The listing builds one solid part. Answer for the finished solid, in the listing's coordinates (mm). A direction names the side the tool comes from. Coordinates: 2 decimals unless noted, no trailing zeros. Order: outer loops, then holes, each group sorted by start corner. A loop starts at its lowest first (then second) coordinate and runs counter-clockwise, first axis right, second up. Notation, with made-up numbers: (52.25, 6.5) -> (70.25, 6.5) arc R21 cw to (70.25, 36.5) -> close; hole circle Ø5 at (-13.5, 32.25). An arc over 180 degrees is marked (long way). Return JSON: item names as keys, results as strings.
```python
from build123d import *
from build123d.topology import SkipClean

# Parameters (mm, degrees)
SALIENTE_EXTRUIR1_DEPTH = 2
SALIENTE_EXTRUIR2_DEPTH = 6.5
SALIENTE_EXTRUIR4_DEPTH = 2.4
SALIENTE_EXTRUIR5_START = 2.4
SALIENTE_EXTRUIR5_DEPTH = 0.9
REDONDEO1_R             = 3
CROQUIS8_W              = 0.8
CROQUIS8_H              = 20.7
SALIENTE_EXTRUIR6_DEPTH = 1.5
CROQUIS9_W              = 18
CROQUIS9_H              = 18
CORTAR_EXTRUIR1_DEPTH   = 2
REDONDEO2_R             = 1


with BuildPart() as part:
    # Croquis1 → Saliente-Extruir1 (new body)
    with BuildSketch(Plane.XY):
        with BuildLine():
            Line((-198.83724752, 71.433656958), (-144.63724752, 71.433656958))
            Line((-144.63724752, 71.433656958), (-144.63724752, 79.683656958))
            ThreePointArc((-144.63724752, 79.683656958), (-139.157169966, 81.953579404), (-136.88724752, 87.433656958))
            Line((-136.88724752, 87.433656958), (-136.88724752, 108.133656958))
            ThreePointArc((-136.88724752, 108.133656958), (-139.157169966, 113.613734512), (-144.63724752, 115.883656958))
            Line((-144.63724752, 115.883656958), (-168.63724752, 115.883656958))
            ThreePointArc((-168.63724752, 115.883656958), (-174.117325074, 113.613734512), (-176.38724752, 108.133656958))
            Line((-176.38724752, 108.133656958), (-198.83724752, 108.133656958))
            Line((-198.83724752, 108.133656958), (-198.83724752, 71.433656958))
        make_face()
        with BuildLine():
            Line((-144.63724752, 83.433656958), (-168.63724752, 83.433656958))
            ThreePointArc((-168.63724752, 83.433656958), (-171.465674645, 84.605229833), (-172.63724752, 87.433656958))
            Line((-172.63724752, 87.433656958), (-172.63724752, 108.133656958))
            ThreePointArc((-172.63724752, 108.133656958), (-171.465674645, 110.962084083), (-168.63724752, 112.133656958))
            Line((-168.63724752, 112.133656958), (-144.63724752, 112.133656958))
            ThreePointArc((-144.63724752, 112.133656958), (-141.808820395, 110.962084083), (-140.63724752, 108.133656958))
            Line((-140.63724752, 108.133656958), (-140.63724752, 87.433656958))
            ThreePointArc((-140.63724752, 87.433656958), (-141.808820395, 84.605229833), (-144.63724752, 83.433656958))
        make_face(mode=Mode.SUBTRACT)
    extrude(amount=SALIENTE_EXTRUIR1_DEPTH)

    # Croquis3 → Saliente-Extruir2 (add)
    with BuildSketch(Plane.XY.offset(2)):
        with BuildLine():
            Line((-136.88724752, 87.433656958), (-136.88724752, 108.133656958))
            ThreePointArc((-136.88724752, 108.133656958), (-139.157169966, 113.613734512), (-144.63724752, 115.883656958))
            Line((-144.63724752, 115.883656958), (-168.63724752, 115.883656958))
            ThreePointArc((-168.63724752, 115.883656958), (-174.117325074, 113.613734512), (-176.38724752, 108.133656958))
            Line((-176.38724752, 108.133656958), (-176.38724752, 87.433656958))
            ThreePointArc((-176.38724752, 87.433656958), (-174.117325074, 81.953579404), (-168.63724752, 79.683656958))
            Line((-168.63724752, 79.683656958), (-144.63724752, 79.683656958))
            ThreePointArc((-144.63724752, 79.683656958), (-139.157169966, 81.953579404), (-136.88724752, 87.433656958))
        make_face()
        with BuildLine():
            Line((-140.63724752, 87.433656958), (-140.63724752, 108.133656958))
            ThreePointArc((-140.63724752, 108.133656958), (-141.808820395, 110.962084083), (-144.63724752, 112.133656958))
            Line((-144.63724752, 112.133656958), (-168.63724752, 112.133656958))
            ThreePointArc((-168.63724752, 112.133656958), (-171.465674645, 110.962084083), (-172.63724752, 108.133656958))
            Line((-172.63724752, 108.133656958), (-172.63724752, 87.433656958))
            ThreePointArc((-172.63724752, 87.433656958), (-171.465674645, 84.605229833), (-168.63724752, 83.433656958))
            Line((-168.63724752, 83.433656958), (-144.63724752, 83.433656958))
            ThreePointArc((-144.63724752, 83.433656958), (-141.808820395, 84.605229833), (-140.63724752, 87.433656958))
        make_face(mode=Mode.SUBTRACT)
    extrude(amount=SALIENTE_EXTRUIR2_DEPTH)

    # Croquis6 → Saliente-Extruir4 (add)
    with SkipClean():  # the faces are left unmerged after this step: merging them gives an invalid solid
        with BuildSketch(Plane.XY.offset(8.5)):
            with BuildLine():
                Line((-172.617197268, 114.783656958), (-140.657297772, 114.783656958))
                ThreePointArc((-140.657297772, 114.783656958), (-142.572665238, 115.603596717), (-144.63724752, 115.883656958))
                Line((-144.63724752, 115.883656958), (-168.63724752, 115.883656958))
                ThreePointArc((-168.63724752, 115.883656958), (-170.701829802, 115.603596717), (-172.617197268, 114.783656958))
            make_face()
            with BuildLine():
                Line((-144.63724752, 79.683656958), (-168.63724752, 79.683656958))
                ThreePointArc((-168.63724752, 79.683656958), (-170.701829802, 79.963717199), (-172.617197268, 80.783656958))
                Line((-172.617197268, 80.783656958), (-140.657297772, 80.783656958))
                ThreePointArc((-140.657297772, 80.783656958), (-142.572665238, 79.963717199), (-144.63724752, 79.683656958))
            make_face()
            with BuildLine():
                Line((-174.63724752, 113.039011176), (-174.63724752, 106.133656958))
                Line((-174.63724752, 106.133656958), (-176.38724752, 106.133656958))
                Line((-176.38724752, 106.133656958), (-176.38724752, 108.133656958))
                ThreePointArc((-176.38724752, 108.133656958), (-175.93664818, 110.73774029), (-174.63724752, 113.039011176))
            make_face()
            with BuildLine():
                Line((-176.38724752, 87.433656958), (-176.38724752, 89.433656958))
                Line((-176.38724752, 89.433656958), (-174.63724752, 89.433656958))
                Line((-174.63724752, 89.433656958), (-174.63724752, 82.52830274))
                ThreePointArc((-174.63724752, 82.52830274), (-175.93664818, 84.829573626), (-176.38724752, 87.433656958))
            make_face()
        extrude(amount=SALIENTE_EXTRUIR4_DEPTH)

    # Croquis7 → Saliente-Extruir5 (add)
    with SkipClean():  # the faces are left unmerged after this step: merging them gives an invalid solid
        with BuildSketch(Plane.XY.offset(8.5).offset(SALIENTE_EXTRUIR5_START)):
            with BuildLine():
                Line((-172.78724752, 106.133656958), (-172.78724752, 108.133656958))
                ThreePointArc((-172.78724752, 108.133656958), (-171.571740662, 111.0681501), (-168.63724752, 112.283656958))
                Line((-168.63724752, 112.283656958), (-144.63724752, 112.283656958))
                ThreePointArc((-144.63724752, 112.283656958), (-143.531697008, 112.133689216), (-142.506048622, 111.6946247))
                Line((-142.506048622, 111.6946247), (-140.657297772, 114.783656958))
                ThreePointArc((-140.657297772, 114.783656958), (-142.572665238, 115.603596717), (-144.63724752, 115.883656958))
                Line((-144.63724752, 115.883656958), (-168.63724752, 115.883656958))
                ThreePointArc((-168.63724752, 115.883656958), (-174.117325074, 113.613734512), (-176.38724752, 108.133656958))
                Line((-176.38724752, 108.133656958), (-176.38724752, 106.133656958))
                Line((-176.38724752, 106.133656958), (-172.78724752, 106.133656958))
            make_face()
            with BuildLine():
                Line((-168.63724752, 79.683656958), (-144.63724752, 79.683656958))
                ThreePointArc((-144.63724752, 79.683656958), (-142.572665238, 79.963717199), (-140.657297772, 80.783656958))
                Line((-140.657297772, 80.783656958), (-142.506048622, 83.872689216))
                ThreePointArc((-142.506048622, 83.872689216), (-143.531697008, 83.4336247), (-144.63724752, 83.283656958))
                Line((-144.63724752, 83.283656958), (-168.63724752, 83.283656958))
                ThreePointArc((-168.63724752, 83.283656958), (-171.571740662, 84.499163816), (-172.78724752, 87.433656958))
                Line((-172.78724752, 87.433656958), (-172.78724752, 89.433656958))
                Line((-172.78724752, 89.433656958), (-176.38724752, 89.433656958))
                Line((-176.38724752, 89.433656958), (-176.38724752, 87.433656958))
                ThreePointArc((-176.38724752, 87.433656958), (-174.117325074, 81.953579404), (-168.63724752, 79.683656958))
            make_face()
        extrude(amount=SALIENTE_EXTRUIR5_DEPTH)

    # Redondeo1
    redondeo1_edges = [part.edges().sort_by_distance(p)[0] for p in [
        (-141.808820395, 84.605229833, 0),
        (-140.63724752, 97.783656958, 0),
        (-141.808820395, 110.962084083, 0),
        (-156.63724752, 112.133656958, 0),
        (-171.465674645, 110.962084083, 0),
        (-172.63724752, 97.783656958, 0),
        (-171.465674645, 84.605229833, 0),
        (-156.63724752, 83.433656958, 0),
    ]]
    fillet(redondeo1_edges, radius=REDONDEO1_R)

    # Croquis8 → Saliente-Extruir6 (add)
    with SkipClean():  # the faces are left unmerged after this step: merging them gives an invalid solid
        with BuildSketch(Plane.XY.offset(8.5)):
            with Locations((-137.28724752, 97.783656958)):
                Rectangle(CROQUIS8_W, CROQUIS8_H)
        extrude(amount=SALIENTE_EXTRUIR6_DEPTH)

    # Croquis9 → Cortar-Extruir1 (cut)
    with SkipClean():  # the faces are left unmerged after this step: merging them gives an invalid solid
        with BuildSketch(Plane.XY.offset(2)):
            with Locations((-186.83724752, 94.133656958)):
                Rectangle(CROQUIS9_W, CROQUIS9_H)
        extrude(amount=-CORTAR_EXTRUIR1_DEPTH, mode=Mode.SUBTRACT)

    # Redondeo2
    redondeo2_edges = [part.edges().sort_by_distance(p)[0] for p in [
        (-177.83724752, 85.133656958, 1),
        (-177.83724752, 103.133656958, 1),
        (-195.83724752, 103.133656958, 1),
        (-195.83724752, 85.133656958, 1),
    ]]
    fillet(redondeo2_edges, radius=REDONDEO2_R)


solid = part.part
```
Item 1: The part is cut by section A-A on x = -167.5. Determine the outline of the cut face in (y, z).
Answer list:
{"outline": "(71.43, 0) -> (80.43, 0) arc R3 ccw to (83.43, 3) -> (83.43, 8.5) -> (80.78, 8.5) -> (80.78, 10.9) -> (83.28, 10.9) -> (83.28, 11.8) -> (79.68, 11.8) -> (79.68, 2) -> (71.43, 2) -> close; (112.13, 3) arc R3 ccw to (115.13, 0) -> (115.88, 0) -> (115.88, 11.8) -> (112.28, 11.8) -> (112.28, 10.9) -> (114.78, 10.9) -> (114.78, 8.5) -> (112.13, 8.5) -> close"}
Item 2: The part is cut by section D-D on x = -182.5. Determine the outline of the cut face in (y, z), plus the area to 3 significant figures.
Answer list:
{"outline": "(71.43, 0) -> (85.13, 0) -> (85.13, 2) -> (71.43, 2) -> close; (103.13, 0) -> (108.13, 0) -> (108.13, 2) -> (103.13, 2) -> close", "area": "37.4 mm2"}
Item 3: Flat-ended cylindrical pins translate along their axes: pin 1 (3.5 mm diameter, centred on x = -174.5, z = 10, fed in from +Y); pin 2 (4.5 mm diameter, centred on y = 99.5, z = 7, fed in from -X); pin 3 (8 mm diameter, centred on x = -157.5, y = 85, fed in from -Z); pin 4 (6 mm diameter, centred on x = -145, y = 98, fed in from -Z). Find the tip coordinate at first contact, or state that the pin passes through.
Answer list:
{"pin 1": "y = 114.54", "pin 2": "x = -176.39", "pin 3": "z = 0.05", "pin 4": "through"}
Item 4: Determine the mould class of faces 6 (the flat face through (-141.595, 113.218, 11.344)), 7 (the cylindrical face through (-156.805, 82.578, 0.902)), 8 (the flat face through (-174.637, 86, 10)), 9 (the flat face through (-174.637, 110, 10)) for opening direction Z: pulls with the +Z half, pulls with the -Z half, needs draft (parallel to the pull), parting line crosses it, or undercut.
Answer list:
{"face 6": "needs draft", "face 7": "pulls with the -Z half", "face 8": "undercut", "face 9": "undercut"}
Item 5: Find the intervals of material crossed by probe 1 along Y at (x, z) = (-152.5, 9.25); probe 2 along X at (y, z) = (88.5, 7); probe 3 along Y at (x, z) = (-147.5, 4.5), in increasing order.
Answer list:
{"probe 1": "79.68 to 80.78, 114.78 to 115.88", "probe 2": "-176.39 to -172.64, -140.64 to -136.89", "probe 3": "79.68 to 83.43, 112.13 to 115.88"}
Item 6: Which of the six approach directions +Z, -Z, +X, -X, +Y, -Y give full straight-line access (tool end or side, diameter ignored) to faces 1 (the flat face through (-187, 103.134, 1)), 2 (the flat face through (-175, 89.434, 10)), 3 (the cylindrical face through (-139.78, 97.64, 0.9)), 4 (the flat face through (-137.687, 98, 9)), 5 (the flat face through (-161.66, 112.44, 10.9))?
Answer list:
{"face 1": "+Z, -Z", "face 2": "+Z, -X", "face 3": "-Z", "face 4": "+Z, +Y, -Y", "face 5": "+X"}
Item 7: The part is cut by section C-C on y = 98.5. Determine the outline of the cut face in (x, z), plus the area to 3 significant figures.
Answer list:
{"outline": "(-198.84, 0) -> (-195.84, 0) -> (-195.84, 2) -> (-198.84, 2) -> close; (-177.84, 0) -> (-175.64, 0) arc R3 ccw to (-172.64, 3) -> (-172.64, 8.5) -> (-176.39, 8.5) -> (-176.39, 2) -> (-177.84, 2) -> close; (-140.64, 3) arc R3 ccw to (-137.64, 0) -> (-136.89, 0) -> (-136.89, 10) -> (-137.69, 10) -> (-137.69, 8.5) -> (-140.64, 8.5) -> close", "area": "70.0 mm2"}
Item 8: The part is cut by section B-B on z = 6.25. Determine the outline of the cut face in (x, y), plus the area to 3 significant figures.
Answer list:
{"outline": "(-176.39, 87.43) arc R7.75 ccw to (-168.64, 79.68) -> (-144.64, 79.68) arc R7.75 ccw to (-136.89, 87.43) -> (-136.89, 108.13) arc R7.75 ccw to (-144.64, 115.88) -> (-168.64, 115.88) arc R7.75 ccw to (-176.39, 108.13) -> close; hole (-172.64, 87.43) arc R4 ccw to (-168.64, 83.43) -> (-144.64, 83.43) arc R4 ccw to (-140.64, 87.43) -> (-140.64, 108.13) arc R4 ccw to (-144.64, 112.13) -> (-168.64, 112.13) arc R4 ccw to (-172.64, 108.13) -> close", "area": "474 mm2"}
